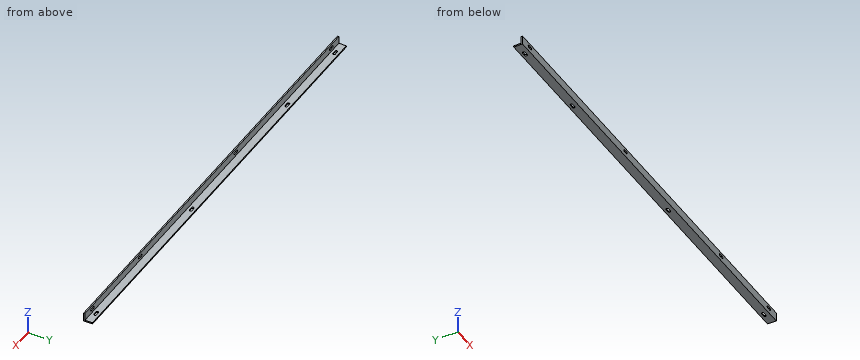
```python
from build123d import *

# Parameters (mm, degrees)
F1_DEPTH = 1020
F3_DEPTH = 3
F5_DEPTH = 3


with BuildPart() as f1:
    # F0 (on Right) → F1 (new body)
    with BuildSketch(Plane.YZ):
        Polygon((0, 20), (0, 0), (20, 0), (20, 3), (3, 3), (3, 20), align=None)
    extrude(amount=F1_DEPTH)

    # F2 (on face) → F3 (cut)
    with BuildSketch(Plane(origin=(0, 3, 0), x_dir=(-1, 0, 0), z_dir=(0, 1, 0))):
        with BuildLine():
            Line((-985.75, 14.25), (-994.25, 14.25))
            ThreePointArc((-994.25, 14.25), (-997, 11.5), (-994.25, 8.75))
            Line((-994.25, 8.75), (-985.75, 8.75))
            ThreePointArc((-985.75, 8.75), (-983, 11.5), (-985.75, 14.25))
        make_face()
        with BuildLine():
            Line((-25.75, 14.25), (-34.25, 14.25))
            ThreePointArc((-34.25, 14.25), (-37, 11.5), (-34.25, 8.75))
            Line((-34.25, 8.75), (-25.75, 8.75))
            ThreePointArc((-25.75, 8.75), (-23, 11.5), (-25.75, 14.25))
        make_face()
        with BuildLine():
            Line((-793.75, 14.25), (-802.25, 14.25))
            ThreePointArc((-802.25, 14.25), (-805, 11.5), (-802.25, 8.75))
            Line((-802.25, 8.75), (-793.75, 8.75))
            ThreePointArc((-793.75, 8.75), (-791, 11.5), (-793.75, 14.25))
        make_face()
        with BuildLine():
            Line((-409.75, 14.25), (-418.25, 14.25))
            ThreePointArc((-418.25, 14.25), (-421, 11.5), (-418.25, 8.75))
            Line((-418.25, 8.75), (-409.75, 8.75))
            ThreePointArc((-409.75, 8.75), (-407, 11.5), (-409.75, 14.25))
        make_face()
    extrude(amount=-F3_DEPTH, mode=Mode.SUBTRACT)

    # F4 (on face) → F5 (cut)
    with BuildSketch(Plane.XY.offset(3)):
        with BuildLine():
            Line((994.25, 14.25), (985.75, 14.25))
            ThreePointArc((985.75, 14.25), (983, 11.5), (985.75, 8.75))
            Line((985.75, 8.75), (994.25, 8.75))
            ThreePointArc((994.25, 8.75), (997, 11.5), (994.25, 14.25))
        make_face()
        with BuildLine():
            Line((226.25, 14.25), (217.75, 14.25))
            ThreePointArc((217.75, 14.25), (215, 11.5), (217.75, 8.75))
            Line((217.75, 8.75), (226.25, 8.75))
            ThreePointArc((226.25, 8.75), (229, 11.5), (226.25, 14.25))
        make_face()
        with BuildLine():
            Line((34.25, 14.25), (25.75, 14.25))
            ThreePointArc((25.75, 14.25), (23, 11.5), (25.75, 8.75))
            Line((25.75, 8.75), (34.25, 8.75))
            ThreePointArc((34.25, 8.75), (37, 11.5), (34.25, 14.25))
        make_face()
        with BuildLine():
            Line((610.25, 14.25), (601.75, 14.25))
            ThreePointArc((601.75, 14.25), (599, 11.5), (601.75, 8.75))
            Line((601.75, 8.75), (610.25, 8.75))
            ThreePointArc((610.25, 8.75), (613, 11.5), (610.25, 14.25))
        make_face()
    extrude(amount=-F5_DEPTH, mode=Mode.SUBTRACT)


solid = f1.part
```
Input: part model. Units: mm. Frame: model coordinates. Give positions to 0.01 mm unless a question says otherwise; leave off trailing zeros. Order: outer loops, then holes, each group sorted by start corner. A loop starts at its lowest first (then second) coordinate and runs counter-clockwise, first axis right, second up. Notation, with made-up numbers: (27.5, 85.25) - (39.5, 85.25) arc R14 ccw to (39.5, 103.25) - close; hole circle Ø6 at (45.25, -22). An arc over 180 degrees is marked (long way). Put each result on its own line as item: value.
Item 1: Contact query for flat-ended pins moving along their axis: pin 1 (5 mm diameter, centred on x = 650.5, y = 15, fed in from +Z); pin 2 (2 mm diameter, centred on x = 224.5, z = 10, fed in from +Y). Output: stop coordinate, or through.
Found:
pin 1: stops at z = 3
pin 2: stops at y = 3
Item 2: Ray query, L1, parallel to Y at x = 292, z = 11. Return the intervals inside material, ascending. Write a range as from..to.
Found:
L1: y = 0..3
Item 3: Section query A-A, the plane x = 117.5. Return loops of the section in (y, z).
Found:
outline: (0, 0) - (20, 0) - (20, 3) - (3, 3) - (3, 20) - (0, 20) - close
